from build123d import *

# Parameters (mm, degrees)
SKETCH1_W           = 80
SKETCH1_H           = 20
BOSS_EXTRUDE1_DEPTH = 3
SKETCH2_R           = 1.5
CUT_EXTRUDE1_DEPTH  = 6
CUT_EXTRUDE2_DEPTH  = 3


with BuildPart() as part:
    # Sketch1 → Boss-Extrude1 (new body)
    with BuildSketch(Plane.XY):
        with Locations((40, 10)):
            Rectangle(SKETCH1_W, SKETCH1_H)
    extrude(amount=BOSS_EXTRUDE1_DEPTH)

    # Sketch2 → Cut-Extrude1 (cut)
    with BuildSketch(Plane(origin=(88.772654641, -6.468882819, 0), x_dir=(-1, 0, 0), z_dir=(0, 0, -1))):
        with Locations((16.772654641, 11.468882819)):
            Circle(SKETCH2_R)
        with Locations((48.772654641, 11.468882819)):
            Circle(SKETCH2_R)
        with Locations((80.772654641, 11.468882819)):
            Circle(SKETCH2_R)
    extrude(amount=-CUT_EXTRUDE1_DEPTH, mode=Mode.SUBTRACT)

    # Sketch3 → Cut-Extrude2 (cut)
    with BuildSketch(Plane(origin=(88.772654641, -6.468882819, 0), x_dir=(-1, 0, 0), z_dir=(0, 0, -1))):
        with BuildLine():
            Line((46.522654641, 23.968882819), (47.095603657, 23.968882819))
            ThreePointArc((47.095603657, 23.968882819), (50.522654641, 23.468882819), (47.095603657, 22.968882819))
            Line((47.095603657, 22.968882819), (46.522654641, 22.968882819))
            Line((46.522654641, 22.968882819), (46.522654641, 23.968882819))
        make_face()
    extrude(amount=-CUT_EXTRUDE2_DEPTH, mode=Mode.SUBTRACT)


solid = part.part
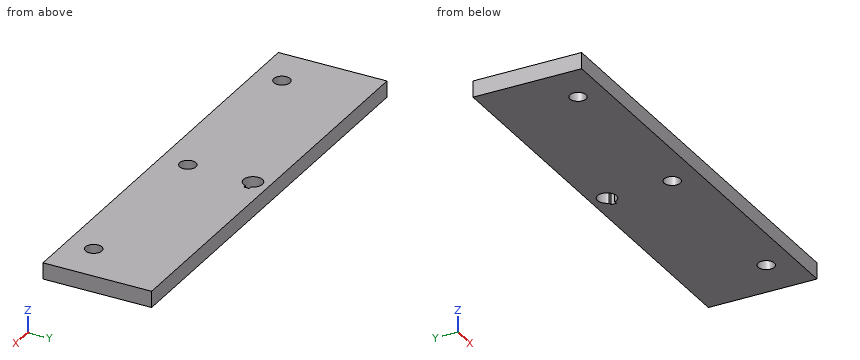
Source: CAD feature listing. Evaluate the final solid. Frame: model axes, mm. Round coordinates to 2 decimals unless told otherwise and drop trailing zeros. Loops run counter-clockwise (first coordinate to the right, second up) from the corner with the lowest first, then second, coordinate; pieces in that order, holes last. Notation, with made-up numbers: M -29,-11.5 L -24,-11.5 A23 cw -24,17.5 Z; hole C 48.5,24.25 d6. An arc over 180 degrees is marked long. Return JSON: item names as keys, results as strings. Group by question number.
1. Section query C-C on x = 40. Output: boundary loops of the cut face in (y, z), and give its area (3 significant figures).
2. Section query A-A on x = 8. Output: boundary loops of the cut face in (y, z), and give its area (3 significant figures).
3. Section query D-D on y = 5. Output: boundary loops of the cut face in (x, z).
4. Material intervals for line 1 along X through (y, z) = (17, 2.3); line 2 along Y through (x, z) = (8, 1.2); line 3 along X through (y, z) = (4.25, 0.25), sorted ascending. Write a range as from..to.
5. Section query B-B on z = 2.4. Output: boundary loops of the cut face in (x, y), and give its area (3 significant figures).
Checks:
{
 "1": {"outline": "M 0,0 L 3.5,0 L 3.5,3 L 0,3 Z; M 6.5,0 L 15.25,0 L 15.25,3 L 6.5,3 Z; M 18.75,0 L 20,0 L 20,3 L 18.75,3 Z", "area": "40.5 mm²"},
 "2": {"outline": "M 0,0 L 3.5,0 L 3.5,3 L 0,3 Z; M 6.5,0 L 20,0 L 20,3 L 6.5,3 Z", "area": "51.0 mm²"},
 "3": {"outline": "M 0,0 L 6.5,0 L 6.5,3 L 0,3 Z; M 9.5,0 L 38.5,0 L 38.5,3 L 9.5,3 Z; M 41.5,0 L 70.5,0 L 70.5,3 L 41.5,3 Z; M 73.5,0 L 80,0 L 80,3 L 73.5,3 Z"},
 "4": {"line 1": "x = 0..38.25, 42.25..80", "line 2": "y = 0..3.5, 6.5..20", "line 3": "x = 0..6.7, 9.3..38.7, 41.3..70.7, 73.3..80"},
 "5": {"outline": "M 0,0 L 80,0 L 80,20 L 0,20 Z; hole C 8,5 d3; hole C 40,5 d3; hole M 41.68,16.5 L 42.25,16.5 L 42.25,17.5 L 41.68,17.5 A1.75 ccw long Z; hole C 72,5 d3", "area": "1,570 mm²"}
}
